For this review, take the finished solid that the model builds, in its own axes (mm). A direction names the side the tool comes from. Coordinates: 2 decimals unless noted, no trailing zeros. Write each loop counter-clockwise with the first axis right and the second up, starting at its lowest first coordinate (ties: lowest second). Pieces come first, ordered by that corner, then holes. Notation, with made-up numbers: M 82.5,2 L 125.5,2 A36 cw 125.5,41 Z; hole C 76,76.5 d5. An arc over 180 degrees is marked long. Return JSON: item names as keys, results as strings.
Autodesk Fusion 360 part; units mm, degrees
sketch "Panel_Dims" plane through (0, 0, 0) normal (0, 0, 1) x (1, 0, 0)
  line L0 (-180, 103.5) -> (180, 103.5) construction
  line L1 (180, 103.5) -> (180, -103.5) construction
  line L2 (180, -103.5) -> (-180, -103.5) construction
  line L3 (-180, -103.5) -> (-180, 103.5) construction
  line L4 (0, 0) -> (0, 103.5) construction
  line L5 (0, 0) -> (-180, 0) construction
  line L6 (-160, -103.5) -> (-160, -111.5)
  line L7 (-145, -103.5) -> (-145, -111.5)
  line L8 (-145, -111.5) -> (-160, -111.5)
  line L9 (-142, -103.5) -> (-142, -114)
  line L10 (160, -103.5) -> (160, -111.5)
  line L11 (145, -103.5) -> (145, -111.5)
  line L12 (160, -111.5) -> (145, -111.5)
  line L13 (139.5, -103.5) -> (139.5, -114)
  line L14 (139.5, -114) -> (-142, -114)
  line L15 (-160, 103.5) -> (-160, 109.8)
  line L16 (-160, 109.8) -> (-147, 109.8)
  line L17 (-147, 109.8) -> (-147, 103.5)
  line L18 (160, 103.5) -> (160, 109.8)
  line L19 (160, 109.8) -> (147, 109.8)
  line L20 (147, 109.8) -> (147, 103.5)
  line L21 (-180, 103.5) -> (-180, -103.5)
  line L22 (-180, -103.5) -> (-160, -103.5)
  line L23 (-145, -103.5) -> (-142, -103.5)
  line L24 (145, -103.5) -> (139.5, -103.5)
  line L25 (160, -103.5) -> (180, -103.5)
  line L26 (180, 103.5) -> (180, -103.5)
  line L27 (-160, 103.5) -> (-180, 103.5)
  line L28 (-147, 103.5) -> (147, 103.5)
  line L29 (160, 103.5) -> (180, 103.5)
  line L30 (-142, -103.5) -> (139.5, -103.5)
  circle A0 centre (-156.5, -106.7) radius 1.2
  circle A1 centre (-148.5, -106.7) radius 1.2
  line L31 (-156.5, -106.7) -> (-148.5, -106.7) construction
  circle A2 centre (148.5, -106.7) radius 1.2
  line L32 (148.5, -106.7) -> (156.5, -106.7) construction
  circle A3 centre (156.5, -106.7) radius 1.2
  circle A4 centre (-156.5, 106.7) radius 1.2
  line L33 (-156.5, 106.7) -> (-150.5, 106.7) construction
  circle A5 centre (-150.5, 106.7) radius 1.2
  circle A6 centre (150.5, 106.7) radius 1.2
  line L34 (150.5, 106.7) -> (156.5, 106.7) construction
  circle A7 centre (156.5, 106.7) radius 1.2
  line L35 (-174.55, 99) -> (169.45, 99)
  line L36 (169.45, 99) -> (169.45, -94)
  line L37 (169.45, -94) -> (-174.55, -94)
  line L38 (-174.55, -94) -> (-174.55, 99)
  line L39 (145, -103.5) -> (160, -103.5)
  line L40 (147, 103.5) -> (160, 103.5)
  line L41 (-147, 103.5) -> (-160, 103.5)
  line L42 (-160, -103.5) -> (-145, -103.5)
  line L43 (-73, -103.5) -> (-43, -103.5)
  line L44 (-43, -103.5) -> (-43, -114)
  line L45 (-43, -114) -> (-73, -114)
  line L46 (-73, -114) -> (-73, -103.5)
  line L47 (-45, -105) -> (-70, -105)
  line L48 (-70, -105) -> (-70, -109)
  line L49 (-70, -109) -> (-45, -109)
  line L50 (-45, -109) -> (-45, -105)
  point P0 (-156.5, -106.7)
  dimension "panel_w" = 360
  dimension "panel_h" = 207
  dimension "ear_indent" = 20
  dimension "ear_bottom_w" = 15
  dimension "ear_bottom_h" = 8
  dimension "pcb_left_indent" = 38
  dimension "d37" = 20
  dimension "d40" = 8
  dimension "pcb_chin_h" = 10.5
  dimension "pcb_chin_w" = 281.5
  dimension "d45" = 20
  dimension "ear_top_h" = 6.3
  dimension "ear_top_w" = 13
  dimension "d48" = 20
  dimension "d49" = 6.3
  dimension "d50" = 13
  dimension "hole_dist_x" = 3.5
  dimension "hole_dia" = 2.4
  dimension "hole_dist_y" = 3.2
  dimension "d54" = 2.4
  dimension "hole_bottom_ipd" = 8
  dimension "d62" = 2.4
  dimension "d63" = 2.4
  dimension "d64" = 8
  dimension "d65" = 3.2
  dimension "d66" = 3.5
  dimension "d67" = 2.4
  dimension "d68" = 2.4
  dimension "hole_top_ipd" = 6
  dimension "d70" = 3.5
  dimension "d72" = 3.2
  dimension "d73" = 2.4
  dimension "d74" = 2.4
  dimension "d75" = 6
  dimension "d76" = 3.5
  dimension "d77" = 3.2
  dimension "bezel_left" = 5.45
  dimension "bezel_top" = 4.5
  dimension "active_w" = 344
  dimension "active_h" = 193
  dimension "d98" = 30
  dimension "d99" = 10.5
  dimension "d100" = 137
  dimension "d101" = 25
  dimension "d102" = 4
  dimension "d103" = 5
  dimension "d104" = 2
extrude "Extrude2" add sketch "Panel_Dims" against normal blind 3.8 from surface at 3.8 contours L9 L14 L30 L46 | L14 L30 L43 L44 L45 L46 | L13 L14 L30 L44 | L47 L48 L49 L50 makes body 1
extrude "Extrude4" add sketch "Panel_Dims" along normal blind 3 separate body contours L35 L36 L37 L38 makes body 2
extrude "Extrude5" add sketch "Panel_Dims" along normal blind 3.8 contours L21 L22 L23 L24 L25 L26 L27 L28 L29 L30 L39 L40 L41 L42 L43 bodies 1 2
extrude "Extrude6" add sketch "Panel_Dims" along normal blind 0.3 from surface at 3 contours L6 L7 L8 L42 | L15 L16 L17 L41 | L18 L19 L20 L40 | L10 L11 L12 L39 bodies 1
extrude "Extrude7" cut sketch "Panel_Dims" along normal blind 1 contours L47 L48 L49 L50 bodies 1
equation "d37 = ear_indent"
equation "d40 = ear_bottom_h"
equation "d45 = ear_indent"
equation "d48 = ear_indent"
equation "d49 = ear_top_h"
equation "d50 = ear_top_w"
equation "d54 = hole_dia"
equation "d62 = hole_dia"
equation "d63 = hole_dia"
equation "d64 = hole_bottom_ipd"
equation "d65 = hole_dist_y"
equation "d66 = hole_dist_x"
equation "d67 = hole_dia"
equation "d68 = hole_dia"
equation "d70 = hole_dist_x"
equation "d72 = hole_dist_y"
equation "d73 = hole_dia"
equation "d74 = hole_dia"
equation "d75 = hole_top_ipd"
equation "d76 = hole_dist_x"
equation "d77 = hole_dist_y"
equation "screen_thicc = panel_thicc - 0,8 mm"
equation "d94 = screen_thicc"
equation "d97 = panel_thicc"
1. We need section B-B (y = 32.5). State the section outline as (x, z) points.
Checks:
{"outline": "M -180,0 L 180,0 L 180,3.8 L 169.45,3.8 L 169.45,3 L -174.55,3 L -174.55,3.8 L -180,3.8 Z"}
2. Clearance check with flat-ended pins moving along their axes: pin 1 Ø1 at (x, z) = (-84.5, 0.5) entering from +Y; pin 2 Ø0.5 at (y, z) = (-106.5, 0.5) entering from -X; pin 3 Ø5 at (x, y) = (155.5, 108) entering from +Z. State where each tip first meets the part, or that it passes through.
Checks:
{"pin 1": "y = 103.5", "pin 2": "x = -142", "pin 3": "z = 3.3"}
3. Wall thickness on L1, parallel to Y at x = 148.5, z = 3.2; L2, parallel to Y at x = -156.5, z = 3.1; L3, parallel to X at y = 106.7, z = 3.1: over which ranges is each line inside the solid? List them lowest first. Write a range as from..to.
Checks:
{"L1": "-111.5..-107.9, -105.5..-94, 99..109.8", "L2": "-111.5..-107.9, -105.5..-94, 99..105.5, 107.9..109.8", "L3": "-160..-157.7, -155.3..-151.7, -149.3..-147, 147..149.3, 151.7..155.3, 157.7..160"}
4. For faces 3 (the face through (-3, -4, 0)), 4 (the face through (39, -101, 3.8)), 5 (the face through (152, -107, 3.3)), 6 (the face through (-153, -107, 3.3)), 7 (the face through (-153, -107, 3)), list the 3-axis set-ups (+Z, -Z, +X, -X, +Y, -Y) from which the entire face can be reached by the end or side of a thin tool; tool diameter is ignored.
Checks:
{"face 3": "-Z, +X, -X, +Y, -Y", "face 4": "+Z, +X, -X, +Y, -Y", "face 5": "+Z, +X, -Y", "face 6": "+Z, -X, -Y", "face 7": "-Z, -X, -Y"}
5. We need section C-C (x = -65). State the section outline as (y, z) points, plus the area to 3 significant figures.
Checks:
{"outline": "M -114,0 L -109,0 L -109,1 L -105,1 L -105,0 L 103.5,0 L 103.5,3.8 L 99,3.8 L 99,3 L -94,3 L -94,3.8 L -114,3.8 Z", "area": "668 mm2"}
6. Draft analysis for pull direction Y (two halves, no side actions). For faces 1 (the face through (-5, 4, 3)), 2 (the face through (152, -107, 3)), state which applies: +Y half, -Y half, draft (parallel to the pull), parting line (faces both ways), or undercut.
Checks:
{"face 1": "undercut", "face 2": "draft"}
7. We need section A-A (x = 131). State the section outline as (y, z) points.
Checks:
{"outline": "M -114,0 L 103.5,0 L 103.5,3.8 L 99,3.8 L 99,3 L -94,3 L -94,3.8 L -114,3.8 Z"}
